from build123d import *

# Parameters (mm, degrees)
ESQUISSE1_W                                 = 44
ESQUISSE1_H                                 = 44
BOSS_EXTRU_1_DEPTH                          = 2
FRAISAGE_POUR_VIS_T_TE_FRAIS_E_M21_AT_COUNT = 2
FRAISAGE_POUR_VIS_T_TE_FRAIS_E_M21_AT_PITCH = 39


with BuildPart() as part:
    # Esquisse1 → Boss.-Extru.1 (new body)
    with BuildSketch(Plane(origin=(0, 0, 0), x_dir=(0, 1, 0), z_dir=(0, 0, 1))):
        Rectangle(ESQUISSE1_W, ESQUISSE1_H)
    extrude(amount=BOSS_EXTRU_1_DEPTH)

    # Esquisse3 → Fraisage pour vis à tête fraisée M21 (revolve, cut)
    with BuildSketch(Plane(origin=(19.5, 19.5, 0), x_dir=(0, 1, 0), z_dir=(1, 0, 0))):
        Polygon((0, 0), (0, 2), (1.2, 2), (1.2, 1), (2.2, 0), align=None)
    fraisage_pour_vis_t_te_frais_e_m21 = revolve(axis=Axis((19.5, 19.5, -6.35), (0, 0, 1)), mode=Mode.SUBTRACT)

    # Fraisage pour vis à tête fraisée M21 at: Fraisage pour vis à tête fraisée M21 ×2
    with Locations(*[(-i * FRAISAGE_POUR_VIS_T_TE_FRAIS_E_M21_AT_PITCH, 0, 0) for i in range(1, FRAISAGE_POUR_VIS_T_TE_FRAIS_E_M21_AT_COUNT)]):
        add(fraisage_pour_vis_t_te_frais_e_m21, mode=Mode.SUBTRACT)

    # Symétrie2: Fraisage pour vis à tête fraisée M21 across plane
    add(fraisage_pour_vis_t_te_frais_e_m21.mirror(Plane.ZX), mode=Mode.SUBTRACT)

    # Symétrie2 copy 1 sketch → Symétrie2 copy 1 (revolve, cut)
    with BuildSketch(Plane(origin=(-19.5, -19.5, 0), x_dir=(0, -1, 0), z_dir=(1, 0, 0))):
        Polygon((0, 0), (0, -2), (1.2, -2), (1.2, -1), (2.2, 0), align=None)
    revolve(axis=Axis((-19.5, -19.5, -6.35), (0, 0, -1)), mode=Mode.SUBTRACT)


solid = part.part
Can you work these out from the model? Positions are in its coordinate system, mm. Coordinates: 2 decimals unless noted, no trailing zeros. Write each loop counter-clockwise with the first axis right and the second up, starting at its lowest first coordinate (ties: lowest second). Pieces come first, ordered by that corner, then holes. Notation, with made-up numbers: (-4.5, 69.5) -> (7.5, 69.5) arc R9 cw to (7.5, 77.5) -> close; hole circle Ø11 at (3.25, 20.25). An arc over 180 degrees is marked (long way). Write each question's results on one line, items separated by ' | '. Start each with the question number.
Q1. We'd pull the mould along X, two halves only. Please class faces 1 (the face through (0, 0, 0)), 2 (the face through (22, 0, 1)), 3 (the face through (20.67, 19.24, 1.49)): +X half, -X half, draft (parallel to the pull), parting line (faces both ways), or undercut.
Q2. Imagine slicing it at A-A (z = 0.3). Write out the boundary of the cut face in (x, y), then the cut area to 3 significant figures.
Q3. I'm going to push flat-ended pins straight in: pin 1 (3 mm diameter, centred on x = 19.5, y = 19.5, fed in from -Z); pin 2 (4 mm diameter, centred on x = 19.5, y = -19.5, fed in from -Z). Where does each tip first touch, or does it pass through?
Q4. Imagine slicing it at B-B (x = -19.5). Write out the boundary of the cut face in (y, z).
Q5. If I drill on probe 1 along Y at (x, z) = (-19.5, 1.5), over which ranges is the centre line in solid material (lowest first)?
Taken from the geometry:
1) face 1: draft | face 2: +X half | face 3: undercut
2) outline: (-22, -22) -> (22, -22) -> (22, 22) -> (-22, 22) -> close; hole circle Ø3.8 at (-19.5, -19.5); hole circle Ø3.8 at (-19.5, 19.5); hole circle Ø3.8 at (19.5, -19.5); hole circle Ø3.8 at (19.5, 19.5) | area: 1,890 mm^2
3) pin 1: stops at z = 0.7 | pin 2: stops at z = 0.2
4) outline: (-22, 0) -> (-21.7, 0) -> (-20.7, 1) -> (-20.7, 2) -> (-22, 2) -> close; (-18.3, 1) -> (-17.3, 0) -> (17.3, 0) -> (18.3, 1) -> (18.3, 2) -> (-18.3, 2) -> close; (20.7, 1) -> (21.7, 0) -> (22, 0) -> (22, 2) -> (20.7, 2) -> close
5) probe 1: y = -22 to -20.7, -18.3 to 18.3, 20.7 to 22
